```python
from build123d import *

# Parameters (mm, degrees)
SKETCH_1_W             = 42
SKETCH_1_H             = 50
BODY_DEPTH             = 0.4
SKETCH_3_R             = 1.35
OLED_PILLAR_DEPTH      = 5
OLED_WINDOW_REACH      = 35.093
SKETCH_2_W             = 30.5
SKETCH_2_H             = 15.5
SKETCH_4_W             = 42
SKETCH_4_H             = 50
SKETCH_4_W_2           = 40
SKETCH_4_H_2           = 48
FARMFEELWALL_DEPTH     = 14
SKETCH_5_W             = 1
SKETCH_5_H             = 42.1
SKETCH_5_H_2           = 48
ESPSUPPORT_DEPTH       = 6
MICRO5PIN_WINDOW_REACH = 52.843
SKETCH_7_W             = 13
SKETCH_7_H             = 6
RESET_WINDOW_REACH     = 58.009
SKETCH_9_W             = 6
SKETCH_9_H             = 4


with BuildPart() as part:
    # 스케치1 → Body (new body)
    with BuildSketch(Plane(origin=(0, 0, 0), x_dir=(1, 0, 0), z_dir=(0, 1, 0))):
        Rectangle(SKETCH_1_W, SKETCH_1_H)
    extrude(amount=BODY_DEPTH)

    # 스케치3 → OLED_pillar (add)
    with BuildSketch(Plane.XZ):
        with Locations(Location((15.25, 14.3, 0), (0, 0, 90))):
            Circle(SKETCH_3_R)
        with Locations(Location((-15.25, -14.3, 0), (0, 0, 90))):
            Circle(SKETCH_3_R)
    extrude(amount=OLED_PILLAR_DEPTH)

    # 스케치2 → OLED_window (cut, up to next)
    with BuildSketch(Plane(origin=(0, 0.4, 0), x_dir=(1, 0, 0), z_dir=(0, 1, 0)), mode=Mode.PRIVATE) as oled_window_sk1:
        with Locations((0, 1.3)):
            Rectangle(SKETCH_2_W, SKETCH_2_H)
    oled_window_tool1 = extrude(oled_window_sk1.sketch, amount=-OLED_WINDOW_REACH, mode=Mode.PRIVATE) & part.part
    add(oled_window_tool1.solids().sort_by_distance((0, 0.4, -1.3))[0], mode=Mode.SUBTRACT)

    # 스케치4 → FarmFeelWall (add)
    with BuildSketch(Plane.XZ):
        Rectangle(SKETCH_4_W, SKETCH_4_H)
        Rectangle(SKETCH_4_W_2, SKETCH_4_H_2, mode=Mode.SUBTRACT)
    extrude(amount=FARMFEELWALL_DEPTH)

    # 스케치5 → EspSupport (add)
    with BuildSketch(Plane.XZ):
        with Locations((-19.5, -2.95)):
            Rectangle(SKETCH_5_W, SKETCH_5_H)
        with Locations((19.5, 0)):
            Rectangle(SKETCH_5_W, SKETCH_5_H_2)
    extrude(amount=ESPSUPPORT_DEPTH)

    # 스케치7 → micro5pin_window (cut, up to next)
    with BuildSketch(Plane.ZY.offset(21), mode=Mode.PRIVATE) as micro5pin_window_sk1:
        with Locations((2.5, -8.5)):
            Rectangle(SKETCH_7_W, SKETCH_7_H)
    micro5pin_window_tool1 = extrude(micro5pin_window_sk1.sketch, amount=-MICRO5PIN_WINDOW_REACH, mode=Mode.PRIVATE) & part.part
    add(micro5pin_window_tool1.solids().sort_by_distance((-21, -8.5, 2.5))[0], mode=Mode.SUBTRACT)

    # 스케치9 → reset_window (cut, up to next)
    with BuildSketch(Plane.XY.offset(25), mode=Mode.PRIVATE) as reset_window_sk1:
        with Locations((-16, -8)):
            Rectangle(SKETCH_9_W, SKETCH_9_H)
    reset_window_tool1 = extrude(reset_window_sk1.sketch, amount=-RESET_WINDOW_REACH, mode=Mode.PRIVATE) & part.part
    add(reset_window_tool1.solids().sort_by_distance((-16, -8, 25))[0], mode=Mode.SUBTRACT)


solid = part.part
```
CAD build for the part. Positions are in the model's coordinates, mm. A direction names the side the tool comes from. Round coordinates to 2 decimals unless told otherwise and drop trailing zeros. Write each loop counter-clockwise with the first axis right and the second up, starting at its lowest first coordinate (ties: lowest second). Pieces come first, ordered by that corner, then holes. Notation, with made-up numbers: M 51,73.25 L 98,73.25 A16 cw 98,82.25 Z; hole C 60.25,65 d7. An arc over 180 degrees is marked long. One line per question, with ' | ' between items.
1. Cut at D-D on z = -20.5. Write the cut outline in (x, y).
Working result:
outline: M -21,-14 L -20,-14 L -20,-6 L -19,-6 L -19,0 L 19,0 L 19,-6 L 20,-6 L 20,-14 L 21,-14 L 21,0.4 L -21,0.4 Z
2. Probe L1, parallel to X at y = -11.5, z = 12.5; L2, parallel to Z at x = 0.5, y = -6.75; L3, parallel to X at y = -5.5, z = -8.5. List the from-to ranges inside material, lowest first. Write a range as from..to.
Working result:
L1: -21..-20, 20..21 | L2: -25..-24, 24..25 | L3: -21..-19, 19..21
3. Cut at B-B on x = 2.5. Write the cut outline in (y, z), and give its area (3 significant figures).
Working result:
outline: M -14,-25 L 0.4,-25 L 0.4,-9.05 L 0,-9.05 L 0,-24 L -14,-24 Z; M -14,24 L 0,24 L 0,6.45 L 0.4,6.45 L 0.4,25 L -14,25 Z | area: 41.8 mm2
4. Mould opens along X. For faces 1 (the flat face through (-21, -5, 0)), 2 (the flat face through (0, -7, -25)), 3 (the cylindrical face through (-15.656, -2.465, -13.012)), 4 (the flat face through (21, -7, 0)) say: pulls with the +X half, pulls with the -X half, needs draft (parallel to the pull), parting line crosses it, or undercut.
Working result:
face 1: pulls with the -X half | face 2: needs draft | face 3: undercut | face 4: pulls with the +X half
5. Cut at A-A on y = -4. Write the cut outline in (x, z), and give its area (3 significant figures).
Working result:
outline: M -21,-25 L 21,-25 L 21,25 L -21,25 Z; C -15.25,-14.3 d2.7; C 15.25,14.3 d2.7; hole M -20,18.1 L -19,18.1 L -19,-24 L 19,-24 L 19,24 L -20,24 Z | area: 282 mm2
6. Cut at C-C on z = 20. Write the cut outline in (x, y), and give its area (3 significant figures).
Working result:
outline: M -21,-14 L -20,-14 L -20,0 L 19,0 L 19,-6 L 20,-6 L 20,-14 L 21,-14 L 21,0.4 L -21,0.4 Z | area: 50.8 mm2
7. Which spindle directions (+Z, -Z, +X, -X, +Y, -Y) get a long thin tool onto all of the face, cutting with end or side? Do faces 5 (the flat face through (-20, -5.5, 2)), 6 (the flat face through (0, -7, 25)), 7 (the flat face through (-20, -12, 0)). Say none if no direction does.
Working result:
face 5: -X | face 6: +Z, +X, -X, +Y, -Y | face 7: -Y
8. Pin check, flat tip, straight feed: pin 1 Ø3 at (x, z) = (-15.5, -13.5) entering from -Y. Stop position of the tip, or through.
Working result:
pin 1: y = -5
